The listing builds one solid part. Answer for the finished solid, in the listing's coordinates (mm). Face numbers are marked on the shaded views. A direction names the side the tool comes from. Round coordinates to 2 decimals unless told otherwise and drop trailing zeros. Write each loop counter-clockwise with the first axis right and the second up, starting at its lowest first coordinate (ties: lowest second). Pieces come first, ordered by that corner, then holes. Notation, with made-up numbers: (44.25, -15) - (62.25, -15) arc R21 ccw to (62.25, 7) - close; hole circle Ø2 at (15, 49). An arc over 180 degrees is marked (long way). Return JSON: item names as keys, results as strings. Group by question number.
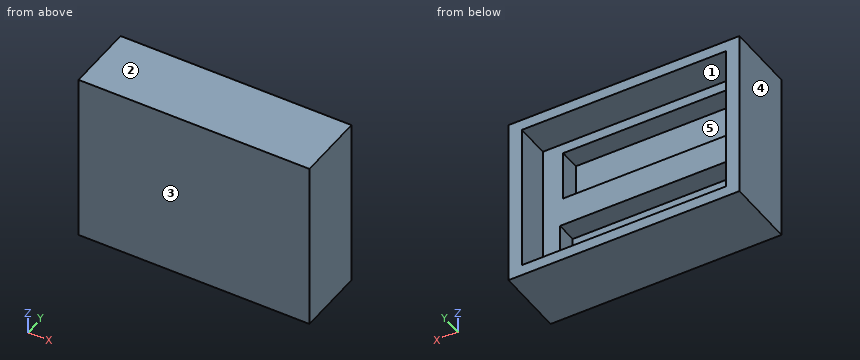
from build123d import *

# Parameters (mm, degrees)
F0_W     = 84.902704
F0_H     = 63.02946
F0_W_2   = 75.117304
F0_H_2   = 54.970898
F0_W_3   = 61.014818
F0_H_3   = 17.843956
F0_W_4   = 60.1514
F0_H_4   = 18.419567
F1_DEPTH = 25.4
F2_DEPTH = 12.7
F3_DEPTH = 20.32


with BuildPart() as f1:
    # F0 (on Front) → F1 (new body)
    with BuildSketch(Plane.XZ):
        Rectangle(F0_W, F0_H)
        Rectangle(F0_W_2, F0_H_2, mode=Mode.SUBTRACT)
        Rectangle(F0_W_2, F0_H_2)
        with Locations((0.719513, -14.246385)):
            Rectangle(F0_W_3, F0_H_3, mode=Mode.SUBTRACT)
        with Locations((-1e-06, 14.53419)):
            Rectangle(F0_W_4, F0_H_4, mode=Mode.SUBTRACT)
        with Locations((-1e-06, 14.53419)):
            Rectangle(F0_W_4, F0_H_4)
        with Locations((0.719513, -14.246385)):
            Rectangle(F0_W_3, F0_H_3)
    extrude(amount=F1_DEPTH)

    # F0 (on Front) → F2 (cut)
    with BuildSketch(Plane.XZ):
        Rectangle(F0_W_2, F0_H_2)
        with Locations((0.719513, -14.246385)):
            Rectangle(F0_W_3, F0_H_3, mode=Mode.SUBTRACT)
        with Locations((-1e-06, 14.53419)):
            Rectangle(F0_W_4, F0_H_4, mode=Mode.SUBTRACT)
        with Locations((-1e-06, 14.53419)):
            Rectangle(F0_W_4, F0_H_4)
        with Locations((0.719513, -14.246385)):
            Rectangle(F0_W_3, F0_H_3)
    extrude(amount=F2_DEPTH, mode=Mode.SUBTRACT)

    # F0 (on Front) → F3 (cut)
    with BuildSketch(Plane.XZ):
        with Locations((-1e-06, 14.53419)):
            Rectangle(F0_W_4, F0_H_4)
        with Locations((0.719513, -14.246385)):
            Rectangle(F0_W_3, F0_H_3)
    extrude(amount=F3_DEPTH, mode=Mode.SUBTRACT)


solid = f1.part
(1) Determine the mould class of the marked faces 1, 2 and 3 for opening direction Z: +Z half, -Z half, draft (parallel to the pull), parting line (faces both ways), or undercut.
(2) For the marked faces 4 and 5, determine the directions among +Z, -Z, +X, -X, +Y, -Y from which every point of the face is accessible in a straight line to the end or side of a thin tool.
(3) Flat-ended cylindrical pins translate along their axes: pin 1 (14.5 mm diameter, centred on x = 1.5, z = -18.5, fed in from +Y); pin 2 (5.5 mm diameter, centred on x = 13, z = 13, fed in from +Y). Find the tip coordinate at first contact, or state that the pin passes through.
(4) Find section D-D (y = -8.5). Write down the section's boundary in (x, z), plus the area to 3 significant figures.
(5) Find section A-A (z = -2.5). Write down the section's boundary in (x, y).
(6) Consider line 1 (Z direction, x = 7, y = -15.5); line 2 (Z direction, x = -28, y = -11); line 3 (X direction, y = -13, z = -16). Determine where each line is inside the solid, lowest interval first.
(7) Find section C-C (y = -15.75). Write down the section's boundary in (x, z), plus the area to 3 significant figures.
(8) Find section B-B (x = -36). Write down the section's boundary in (y, z), plus the area to 3 significant figures.
Check sheet entries:
{
 "1": {"face 1": "undercut", "face 2": "+Z half", "face 3": "draft"},
 "2": {"face 4": "+Z, -Z, -X, +Y, -Y", "face 5": "+Y"},
 "3": {"pin 1": "stops at y = -12.7", "pin 2": "stops at y = -20.32"},
 "4": {"outline": "(-42.45, -31.51) - (42.45, -31.51) - (42.45, 31.51) - (-42.45, 31.51) - close; hole (-37.56, -27.49) - (37.56, -27.49) - (37.56, 27.49) - (-37.56, 27.49) - close", "area": "1,220 mm^2"},
 "5": {"outline": "(-42.45, -25.4) - (42.45, -25.4) - (42.45, 0) - (37.56, 0) - (37.56, -12.7) - (-37.56, -12.7) - (-37.56, 0) - (-42.45, 0) - close"},
 "6": {"line 1": "z = -31.51 to -23.17, -5.32 to 5.32, 23.74 to 31.51", "line 2": "z = -31.51 to -27.49, 27.49 to 31.51", "line 3": "x = -42.45 to -29.79, 31.23 to 42.45"},
 "7": {"outline": "(-42.45, -31.51) - (42.45, -31.51) - (42.45, 31.51) - (-42.45, 31.51) - close; hole (-30.08, 5.32) - (30.08, 5.32) - (30.08, 23.74) - (-30.08, 23.74) - close; hole (-29.79, -23.17) - (31.23, -23.17) - (31.23, -5.32) - (-29.79, -5.32) - close", "area": "3,150 mm^2"},
 "8": {"outline": "(-25.4, -31.51) - (0, -31.51) - (0, -27.49) - (-12.7, -27.49) - (-12.7, 27.49) - (0, 27.49) - (0, 31.51) - (-25.4, 31.51) - close", "area": "903 mm^2"}
}
